from build123d import *

# Parameters (mm, degrees)
SKETCH_1_R      = 1.65
EXTRUDE_2_DEPTH = 3.5
CHAMFER_1_SIZE  = 0.5


with BuildPart() as part:
    # 草图1 → 凸台-拉伸2 (new body)
    with BuildSketch(Plane.XY):
        with BuildLine():
            add(Edge.make_bspline(
                [(-2, 2.236067977), (1.298350605, 5.186202444), (7.70496537, 6.630470955), (13.291718654, 5.552855645), (17, 2.236067977)],
                knots=[0, 0, 0, 0, 0.5, 1, 1, 1, 1], degree=3))
            ThreePointArc((-2, 2.236067977), (-2.236067977, -2), (2, -2.236067977))
            add(Edge.make_bspline(
                [(2, -2.236067977), (2.133231621, -2.116901993), (2.413155894, -1.87779666), (2.92891001, -1.478504787), (3.538329614, -1.07495841), (4.2139596, -0.719034821), (5.07558679, -0.368617139), (5.940240482, -0.155045102), (6.888643765, -0.035603913), (7.691648693, 0.010168459), (8.44481537, 0.011741207), (9.02314593, -0.033114067), (9.5178697, -0.118274629), (9.991466761, -0.252962594), (10.526142012, -0.471507355), (11.180937128, -0.827124358), (11.86067581, -1.292530825), (12.478348447, -1.781196), (12.832651532, -2.086386958), (13, -2.236067977)],
                knots=[0, 0, 0, 0, 0.03125, 0.0625, 0.125, 0.1875, 0.25, 0.375, 0.4375, 0.5, 0.5625, 0.625, 0.6875, 0.75, 0.8125, 0.875, 0.9375, 0.96875, 1, 1, 1, 1], degree=3))
            ThreePointArc((13, -2.236067977), (17.236067977, -2), (17, 2.236067977))
        make_face()
        Circle(SKETCH_1_R, mode=Mode.SUBTRACT)
        with Locations((15, 0)):
            Circle(SKETCH_1_R, mode=Mode.SUBTRACT)
    extrude(amount=EXTRUDE_2_DEPTH)

    # 倒角1
    chamfer_1_edges = [part.edges().sort_by_distance(p)[0] for p in [
        (17.236067977, -2, 0),
        (7.532671852, -0.002579069, 0),
        (-2.236067977, -2, 0),
        (7.532671852, -0.002579069, 0),
    ]]
    chamfer(chamfer_1_edges, length=CHAMFER_1_SIZE)


solid = part.part
Geometry check sheet. Reference: the model listing, model coordinates, mm. Round coordinates to 2 decimals unless told otherwise and drop trailing zeros. One line per item, written item: value. Start each with the question number.
(1) Go/stop test with a flat-tipped pin: pin 1 Ø1.5 at (x, z) = (3.5, 0.5) entering from -Y. Record where the tip stops, or that it passes through.
(2) Cross-section at A-A, the plane z = 1.3. Give the number of separate pieces and of enclosed holes in the cut face, and give its area (3 significant figures).
(3) Draft check along Y on faces 1 (the cylindrical face through (-2.28, -1.95, 1.98)), 2 (the cylindrical face through (-1.216, 1.115, 1.726)), 3 (the flat face through (8, 2, 0)). Enter one of: +Y half, -Y half, draft (parallel to the pull), parting line (faces both ways), or undercut.
(4) Scan lines: line 1 (Y direction, x = -2, z = 1.65); line 2 (X direction, y = 0.5, z = 2.85); line 3 (X direction, y = -1, z = 0.7). Record each from-to range of solid material in increasing order. Write a range as [from, to].
Answer:
1. pin 1: y = -1.62
2. separate pieces: 1
2. enclosed holes: 2
2. area: 111 mm²
3. face 1: parting line
3. face 2: undercut
3. face 3: draft
4. line 1: [-2.24, 2.24]
4. line 2: [-2.96, -1.57], [1.57, 13.43], [16.57, 17.96]
4. line 3: [-2.83, -1.31], [1.31, 3.69], [11.42, 13.69], [16.31, 17.83]
